Part print with two shaded views. Sizes in mm from the minimum x, y, z corner. Give positions to 0.01 mm unless a question says otherwise; leave off trailing zeros. Order: outer loops, then holes, each group sorted by start corner. A loop starts at its lowest first (then second) coordinate and runs counter-clockwise, first axis right, second up. Notation, with made-up numbers: M 31.25,16 L 39.25,16 A17 cw 39.25,38 Z; hole C 24.25,17.25 d5. An arc over 180 degrees is marked long. Return JSON: item names as keys, results as strings. Group by question number.
1. Slice it at B-B on y = 29. List the corners of the cut face in (x, z).
2. Pin check, flat tip, straight feed: pin 1 (2 mm diameter, centred on x = 68, z = 1, fed in from +Y). Stop position of the tip, or through.
3. Slice it at A-A on x = 77.5. List the corners of the cut face in (y, z), then the cut area to 3 significant figures.
4. Wall check: probe 1 along X at (y, z) = (24.5, 3.75); probe 2 along Y at (x, z) = (22, 6); probe 3 along Y at (x, z) = (31, 7.75) (1 decimal). Give the ranges that are in metal, low to high. Write a range as [from, to].
5. Slice it at C-C on z = 4.75. List the corners of the cut face in (x, y).
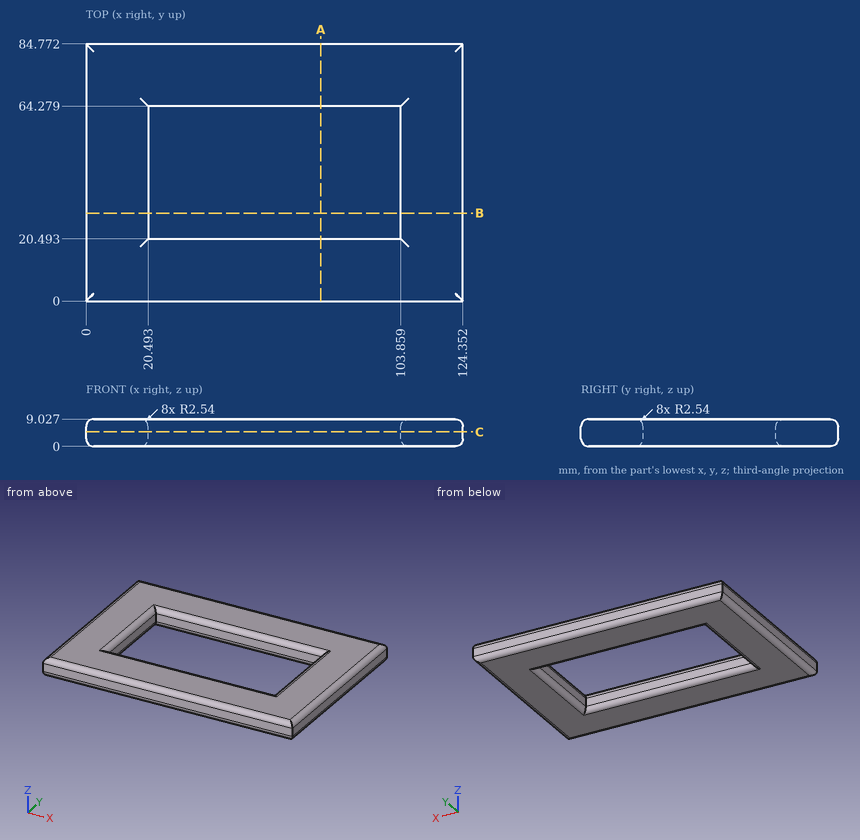
Result:
{
 "1": {"outline": "M 0,2.54 A2.54 ccw 2.54,0 L 17.95,0 A2.54 ccw 20.49,2.54 L 20.49,6.49 A2.54 ccw 17.95,9.03 L 2.54,9.03 A2.54 ccw 0,6.49 Z; M 103.86,2.54 A2.54 ccw 106.4,0 L 121.81,0 A2.54 ccw 124.35,2.54 L 124.35,6.49 A2.54 ccw 121.81,9.03 L 106.4,9.03 A2.54 ccw 103.86,6.49 Z"},
 "2": {"pin 1": "stops at y = 84.71"},
 "3": {"outline": "M 0,2.54 A2.54 ccw 2.54,0 L 17.95,0 A2.54 ccw 20.49,2.54 L 20.49,6.49 A2.54 ccw 17.95,9.03 L 2.54,9.03 A2.54 ccw 0,6.49 Z; M 64.28,2.54 A2.54 ccw 66.82,0 L 82.23,0 A2.54 ccw 84.77,2.54 L 84.77,6.49 A2.54 ccw 82.23,9.03 L 66.82,9.03 A2.54 ccw 64.28,6.49 Z", "area": "359 mm2"},
 "4": {"probe 1": "x = [0, 20.49], [103.86, 124.35]", "probe 2": "y = [0, 20.49], [64.28, 84.77]", "probe 3": "y = [0.3, 20.2], [64.6, 84.4]"},
 "5": {"outline": "M 0,0 L 124.35,0 L 124.35,84.77 L 0,84.77 Z; hole M 20.49,20.49 L 103.86,20.49 L 103.86,64.28 L 20.49,64.28 Z"}
}
